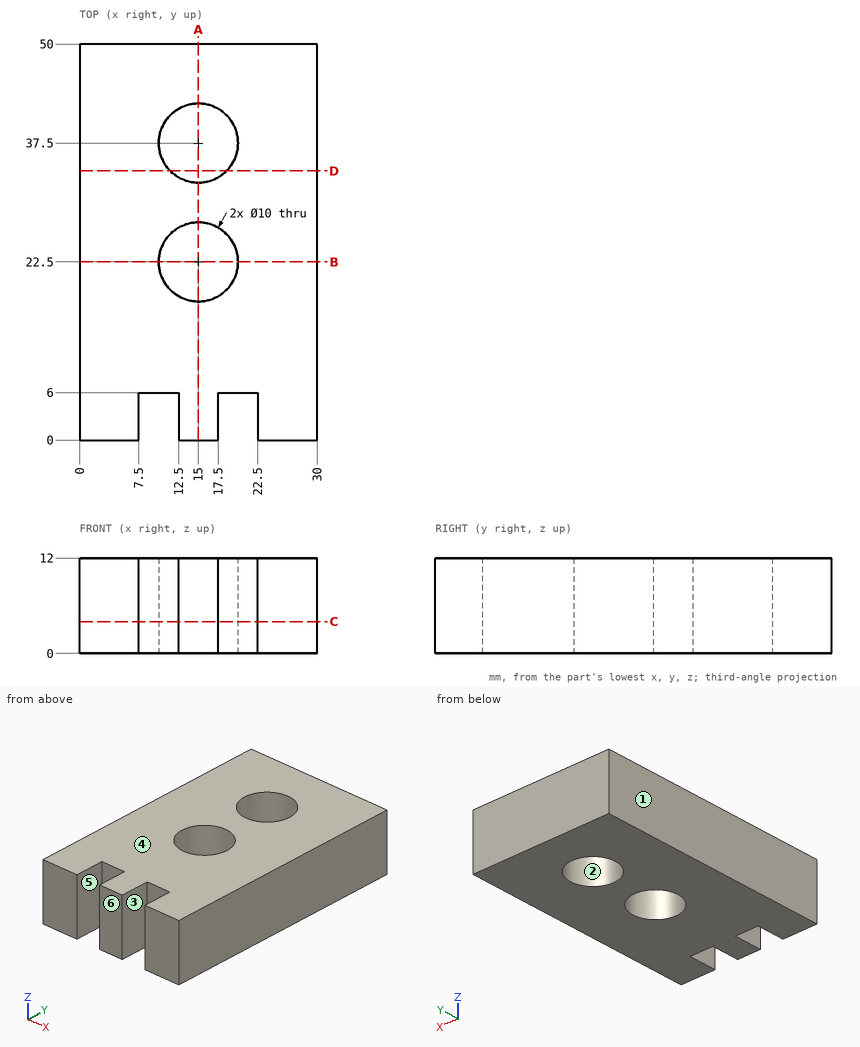
Print and shaded views of the part. All mm, measured from the part's lowest x, y and z. A direction names the side the tool comes from. Give positions to 0.01 mm unless a question says otherwise; leave off trailing zeros. Write each loop counter-clockwise with the first axis right and the second up, starting at its lowest first coordinate (ties: lowest second). Pieces come first, ordered by that corner, then holes. Notation, with made-up numbers: (-1.5, 57.5) -> (34.5, 57.5) arc R21 ccw to (34.5, 71.5) -> close; hole circle Ø5 at (15.25, 24.5). An arc over 180 degrees is marked (long way). Write item = value, one per line.
(1) Slice it at A-A, the plane x = 15. Give the cut face in (y, z), then the cut area to 3 significant figures.
Determined:
outline = (0, 0) -> (17.5, 0) -> (17.5, 12) -> (0, 12) -> close; (27.5, 0) -> (32.5, 0) -> (32.5, 12) -> (27.5, 12) -> close; (42.5, 0) -> (50, 0) -> (50, 12) -> (42.5, 12) -> close
area = 360 mm2
(2) Slice it at C-C, the plane z = 4. Give the cut face in (x, y).
Determined:
outline = (0, 0) -> (7.5, 0) -> (7.5, 6) -> (12.5, 6) -> (12.5, 0) -> (17.5, 0) -> (17.5, 6) -> (22.5, 6) -> (22.5, 0) -> (30, 0) -> (30, 50) -> (0, 50) -> close; hole circle Ø10 at (15, 22.5); hole circle Ø10 at (15, 37.5)
(3) Flat gauge pin, fed straight in: P1, Ø3, axis at x = 15, y = 5.5, coming from the -Z side. Where does the tip first touch, or does it go through?
Determined:
P1 = 0
(4) Probe line 1 along X through (y, z) = (3, 6); line 2 along Y through (x, z) = (15, 5.25); line 3 along X through (y, z) = (37.5, 3). List the from-to ranges inside material, lowest first.
Determined:
line_1 = 0 to 7.5, 12.5 to 17.5, 22.5 to 30
line_2 = 0 to 17.5, 27.5 to 32.5, 42.5 to 50
line_3 = 0 to 10, 20 to 30
(5) Tool access for the marked faces 5 and 6: list every direction of +Z, -Z, +X, -X, +Y, -Y with a clear straight run to the whole face (end or side of a thin tool).
Determined:
face_5 = +Z, -Z, -Y
face_6 = +Z, -Z, +X, -X, -Y
(6) Slice it at B-B, the plane y = 22.5. Give the cut face in (x, z).
Determined:
outline = (0, 0) -> (10, 0) -> (10, 12) -> (0, 12) -> close; (20, 0) -> (30, 0) -> (30, 12) -> (20, 12) -> close
(7) Slice it at D-D, the plane y = 34. Give the cut face in (x, z), then the cut area to 3 significant figures.
Determined:
outline = (0, 0) -> (11.43, 0) -> (11.43, 12) -> (0, 12) -> close; (18.57, 0) -> (30, 0) -> (30, 12) -> (18.57, 12) -> close
area = 274 mm2
(8) Mould opens along X. For the marked faces 1, 2, 3 and 4 say: released by +X, released by -X, zero draft, split by the parting line, or undercut.
Determined:
face_1 = released by -X
face_2 = undercut
face_3 = undercut
face_4 = zero draft
